Source: CAD feature listing. Evaluate the final solid. Frame: model axes, mm. Round coordinates to 2 decimals unless told otherwise and drop trailing zeros. Loops run counter-clockwise (first coordinate to the right, second up) from the corner with the lowest first, then second, coordinate; pieces in that order, holes last. Notation, with made-up numbers: M 46.5,55.5 L 99.5,55.5 A14 ccw 99.5,59.5 Z; hole C 27,-12 d2. An arc over 180 degrees is marked long. Write each question's results on one line, items separated by ' | '. Start each with the question number.
1. Contact query for a flat-ended pin moving along its axis: pin 1 Ø2.5 at (x, z) = (4, -6.93) entering from +Y. Output: stop coordinate, or through.
2. Section D-D on y = 2. Output: boundary loops of the cut face in (x, z).
3. Section C-C on x = 4.75. Output: boundary loops of the cut face in (y, z), and give its area (3 significant figures).
4. Draft query along Z for faces 1 (the cylindrical face through (2.38, 1.48, 10.74)), 2 (the cylindrical face through (6.522, 1.479, -0.466)), 3 (the cylindrical face through (-2.86, 1.48, -7.98)), 4 (the flat face through (-2.3, 0, -2.3)). Return one class per face: released by +Z, released by -Z, zero draft, split by the parting line, or undercut.
5. Section A-A on x = 0. Output: boundary loops of the cut face in (y, z), and give its area (3 significant figures).
6. Section B-B on z = 0. Output: boundary loops of the cut face in (x, y).
7. Ray query, line 1 (X direction, y = 2.8, z = -6); line 2 (Z direction, x = 4, y = 0.8); line 3 (Z direction, x = 4.25, y = 2.5). Return the intervals inside material, ascending.
Autodesk Inventor part; units mm, degrees
ref_plane "YZ Plane" through (0, 0, 0) normal (1, 0, 0) x (0, 1, 0)
ref_plane "XZ Plane" through (0, 0, 0) normal (0, 1, 0) x (-1, 0, 0)
ref_plane "XY Plane" through (0, 0, 0) normal (0, 0, 1) x (1, 0, 0)
sketch "Sketch1" plane through (0, 0, 0) normal (0, 1, 0) x (-1, 0, 0)
  circle A0 centre (0, 0) radius 11
  circle A1 centre (0, 0) radius 8 construction
  circle A2 centre (8, 0) radius 1.55
  line L0 (0, 0) -> (8, 0) construction
  circle A3 centre (4, 6.9282) radius 1.55
  circle A4 centre (-4, 6.9282) radius 1.55
  circle A5 centre (-8, 0) radius 1.55
  circle A6 centre (-4, -6.9282) radius 1.55
  circle A7 centre (4, -6.9282) radius 1.55
  circle A8 centre (0, 0) radius 3
  dimension "d1" = 16
  dimension "d0" = 22
  dimension "d2" = 3.1
  dimension "d5" = 360
  dimension "d9" = 6
extrude "Extrusion1" add sketch "Sketch1" along normal blind 3
properties part number "FlywheelSpacer" material "PC/ABS Plastic"
Taken from the geometry:
1) pin 1: through
2) outline: C 0,0 d22; hole C -8,0 d3.1; hole C -4,-6.93 d3.1; hole C -4,6.93 d3.1; hole C 0,0 d6; hole C 4,-6.93 d3.1; hole C 4,6.93 d3.1; hole C 8,0 d3.1
3) outline: M 0,-9.92 L 3,-9.92 L 3,-8.28 L 0,-8.28 Z; M 0,-5.57 L 3,-5.57 L 3,5.57 L 0,5.57 Z; M 0,8.28 L 3,8.28 L 3,9.92 L 0,9.92 Z | area: 43.3 mm^2
4) face 1: split by the parting line | face 2: undercut | face 3: undercut | face 4: zero draft
5) outline: M 0,-11 L 3,-11 L 3,-3 L 0,-3 Z; M 0,3 L 3,3 L 3,11 L 0,11 Z | area: 48.0 mm^2
6) outline: M -11,0 L -9.55,0 L -9.55,3 L -11,3 Z; M -6.45,0 L -3,0 L -3,3 L -6.45,3 Z; M 3,0 L 6.45,0 L 6.45,3 L 3,3 Z; M 9.55,0 L 11,0 L 11,3 L 9.55,3 Z
7) line 1: -9.22 to -5.24, -2.76 to 2.76, 5.24 to 9.22 | line 2: -10.25 to -8.48, -5.38 to 5.38, 8.48 to 10.25 | line 3: -10.15 to -8.46, -5.4 to 5.4, 8.46 to 10.15
